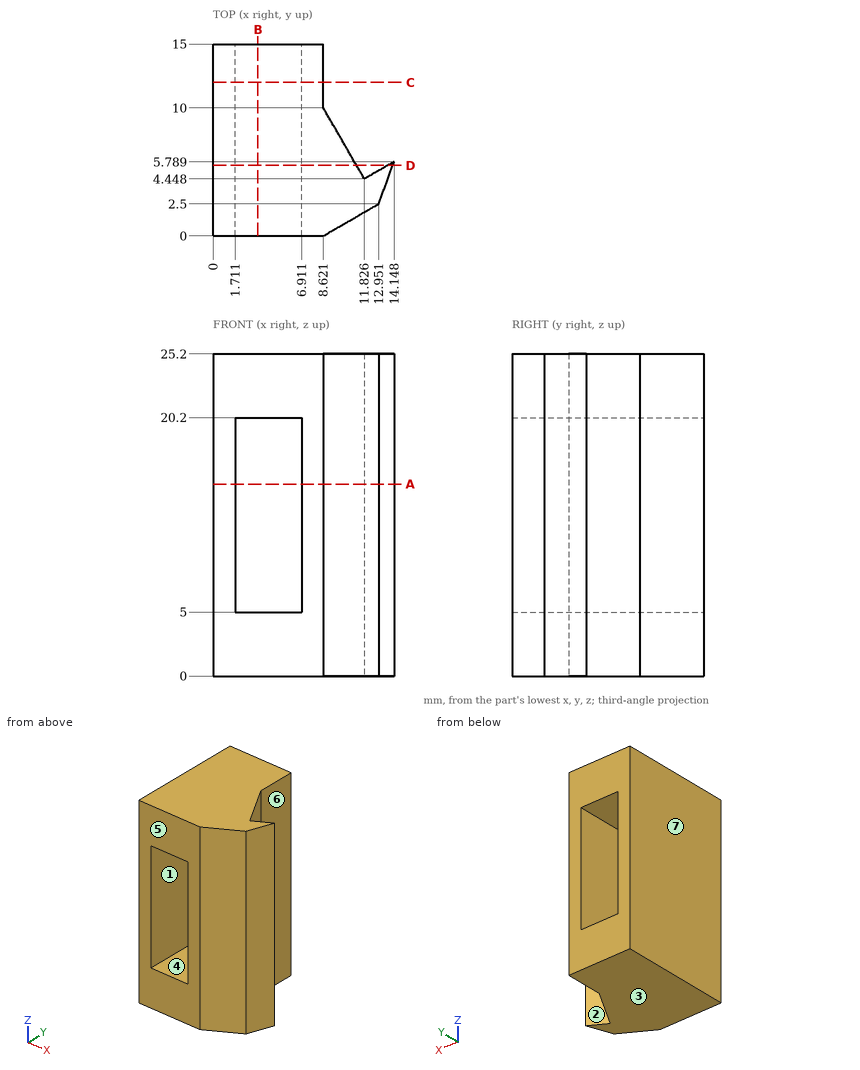
Source: three-view drawing plus pictorial views. Frame: mm from the lowest corner of the part. A direction names the side the tool comes from. Give positions to 0.01 mm unless a question says otherwise; leave off trailing zeros. Loops run counter-clockwise (first coordinate to the right, second up) from the corner with the lowest first, then second, coordinate; pieces in that order, holes last. Notation, with made-up numbers: (60.25, -29.75) -> (103.25, -29.75) arc R29 cw to (103.25, 8.25) -> close; hole circle Ø5 at (-33, 65). An arc over 180 degrees is marked (long way). Put each result on its own line as item: value. Start each with the question number.
1) Cut plane D-D (y = 5.5). Return loops of the section in (x, z).
2) Draft query along X for the marked faces 4, 5, 6 and 7. Return one class per face: released by +X, released by -X, zero draft, split by the parting line, or undercut.
3) Cut plane A-A (z = 15). Return loops of the section in (x, y).
4) Cut plane B-B (x = 3.5). Return loops of the section in (y, z).
5) Cut plane C-C (y = 12). Return loops of the section in (x, z), then the cut area to 3 significant figures.
6) Material intervals for probe 1 along X at (y, z) = (11.5, 16.5); probe 2 along Z at (x, y) = (5.75, 1.5); probe 3 along X at (y, z) = (7, 9.5) (1 decimal), sorted ascending.
7) Reachability of the marked faces 1, 2 and 3 from +Z, -Z, +X, -X, +Y, -Y: full face, straight path, thin tool, end or side. Return the list, or none.
Results are:
1. outline: (0, 0) -> (11.22, 0) -> (11.22, 25.2) -> (0, 25.2) -> close; (13.65, 0) -> (14.04, 0) -> (14.04, 25.2) -> (13.65, 25.2) -> close; hole (1.71, 5) -> (6.91, 5) -> (6.91, 20.2) -> (1.71, 20.2) -> close
2. face 4: undercut
2. face 5: zero draft
2. face 6: released by +X
2. face 7: released by -X
3. outline: (0, 0) -> (1.71, 0) -> (1.71, 15) -> (0, 15) -> close; (6.91, 0) -> (8.62, 0) -> (12.95, 2.5) -> (14.15, 5.79) -> (11.83, 4.45) -> (8.62, 10) -> (8.62, 15) -> (6.91, 15) -> close
4. outline: (0, 0) -> (15, 0) -> (15, 5) -> (0, 5) -> close; (0, 20.2) -> (15, 20.2) -> (15, 25.2) -> (0, 25.2) -> close
5. outline: (0, 0) -> (8.62, 0) -> (8.62, 25.2) -> (0, 25.2) -> close; hole (1.71, 5) -> (6.91, 5) -> (6.91, 20.2) -> (1.71, 20.2) -> close
5. area: 138 mm2
6. probe 1: x = 0 to 1.71, 6.91 to 8.62
6. probe 2: z = 0 to 5, 20.2 to 25.2
6. probe 3: x = 0 to 1.7, 6.9 to 10.4
7. face 1: +Y, -Y
7. face 2: +Z, -Z, +Y
7. face 3: -Z, +X, -X, +Y, -Y
